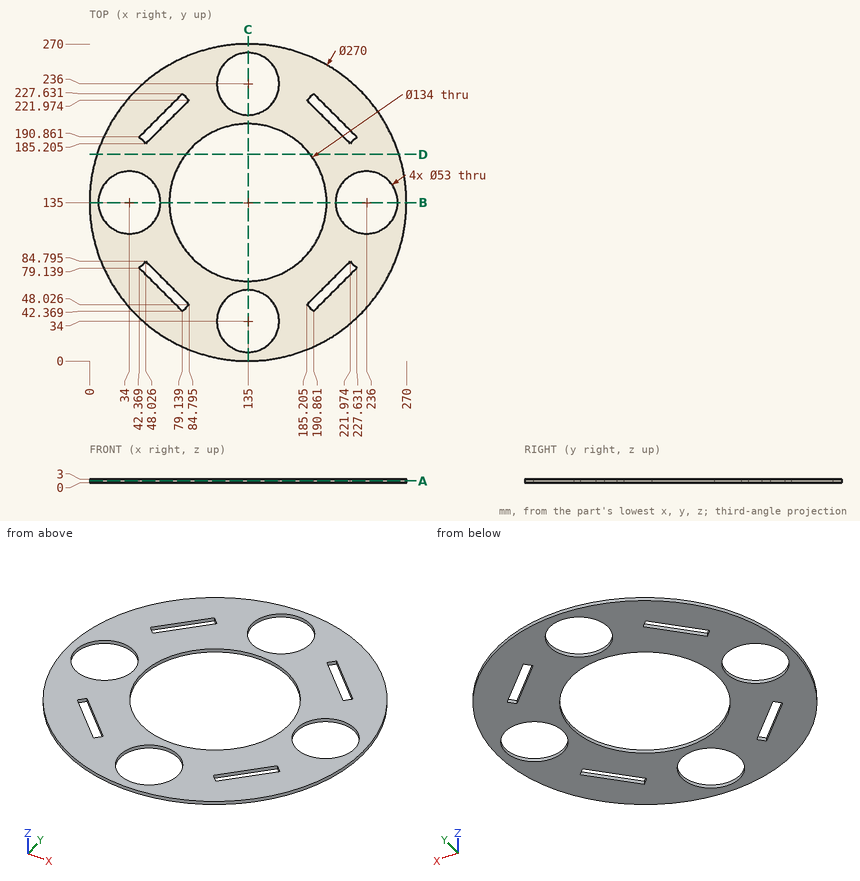
Geometry: see drawing. Coordinates: mm, zero at the bounding-box minimum. Round coordinates to 2 decimals unless told otherwise and drop trailing zeros. Write each loop counter-clockwise with the first axis right and the second up, starting at its lowest first coordinate (ties: lowest second). Pieces come first, ordered by that corner, then holes.
1) Cut plane A-A (z = 1.45). Count the separate pieces of the cut face and the enclosed holes in it, then the cut area to 3 significant figures.
2) Contact query for a flat-ended pin moving along its axis: P1, Ø1, axis at x = 80, z = 1.5, coming from the +Y side. Output: stop coordinate, or through.
3) Cut plane B-B (y = 135). Return the cut outline in (x, z).
4) Cut plane D-D (y = 176). Return the cut outline in (x, z).
5) Ray query, L1, parallel to Y at x = 135, z = 1.2; L2, parallel to X at y = 197, z = 2 (1 decimal); L3, parallel to Y at x = 155, z = 2.65 (1 decimal). Return the intervals inside material, ascending.
Geometry says:
1. separate pieces: 1
1. enclosed holes: 9
1. area: 32,700 mm2
2. P1: stops at y = 258.51
3. outline: (0, 0) - (7.5, 0) - (7.5, 3) - (0, 3) - close; (60.5, 0) - (68, 0) - (68, 3) - (60.5, 3) - close; (202, 0) - (209.5, 0) - (209.5, 3) - (202, 3) - close; (262.5, 0) - (270, 0) - (270, 3) - (262.5, 3) - close
4. outline: (6.38, 0) - (82.01, 0) - (82.01, 3) - (6.38, 3) - close; (187.99, 0) - (263.62, 0) - (263.62, 3) - (187.99, 3) - close
5. L1: y = 0 to 7.5, 60.5 to 68, 202 to 209.5, 262.5 to 270
5. L2: x = 15.1 to 48.5, 59.8 to 109.6, 160.4 to 210.2, 221.5 to 254.9
5. L3: y = 1.5 to 16.6, 51.4 to 71.1, 198.9 to 218.6, 253.4 to 268.5
